Geometry check sheet. Reference: the model listing, model coordinates, mm. A direction names the side the tool comes from. Give positions to 0.01 mm unless a question says otherwise; leave off trailing zeros. Write each loop counter-clockwise with the first axis right and the second up, starting at its lowest first coordinate (ties: lowest second). Pieces come first, ordered by that corner, then holes. Notation, with made-up numbers: (76.5, -36) - (93.5, -36) arc R24 ccw to (93.5, 2) - close; hole circle Ø4 at (75, 0.5). An arc over 180 degrees is marked (long way). One line per question, with ' | ' between items. Start each with the question number.
Q1. Section check C-C on z = 5.75. Record the boundary of the cut face in (x, y) (3 decimals), and give its area (3 significant figures).
Q2. Set-up check for faces 4 (the face through (-33, 19.05, 6)), 5 (the face through (-1, 5, 0)), 6 (the face through (28.575, -4, 6)), 7 (the face through (-5.506, -24.796, 8.004)), 8 (the face through (0, -28.575, 6)): record each of +Z, -Z, +X, -X, +Y, -Y from which the full face is reachable in a straight line by a thin tool's end or side.
Q3. Thickness scan on L1, parallel to Y at x = 0, z = 8.25 (3 decimals); L2, parallel to Z at x = -16, y = 3 (3 decimals); L3, parallel to X at y = -13.5, z = 10 (3 decimals). Record the ranges inside material, lowest first. Write a range as [from, to].
Q4. Section check D-D on x = 32. Record the boundary of the cut face in (y, z), and give its area (3 significant figures).
Q5. Release check for a two-part mould opening along X. For faces 1 (the face through (-1, 27, 12.7)), 2 (the face through (38.1, 28, 6)), 3 (the face through (0, 0, 3.175)) record: +X half, -X half, draft (parallel to the pull), parting line (faces both ways), or undercut.
Q6. Section check B-B on y = 0. Record the boundary of the cut face in (x, z) (3 decimals).
Q7. Section check A-A on x = 0. Record the boundary of the cut face in (y, z) (3 decimals), and give its area (3 significant figures).
Q8. Gauge pin test, flat ends, axial feed: P1, Ø6, axis at y = -2.5, z = 7.5, coming from the +X side (3 decimals); P2, Ø3, axis at x = 33, z = 6, coming from the -Y side; P3, Ø15, axis at x = -0.5, y = -6, coming from the +Z side (3 decimals). Record the tip position at first contact, or that the pin passes through.
```python
from build123d import *

# Parameters (mm, degrees)
SKETCH1_W               = 76.2
SKETCH1_H               = 76.2
BOSS_EXTRUDE1_DEPTH     = 12.7
SKETCH2_R               = 25.4
CUT_EXTRUDE1_DEPTH      = 9.525
CUT_EXTRUDE3_DEPTH      = 1
CUT_EXTRUDE3_DEPTH_BACK = 13.7


with BuildPart() as part:
    # Sketch1 → Boss-Extrude1 (new body)
    with BuildSketch(Plane.XY):
        Rectangle(SKETCH1_W, SKETCH1_H)
    extrude(amount=BOSS_EXTRUDE1_DEPTH)

    # Sketch2 → Cut-Extrude1 (cut)
    with BuildSketch(Plane.XY.offset(12.7)):
        Circle(SKETCH2_R)
    extrude(amount=-CUT_EXTRUDE1_DEPTH, mode=Mode.SUBTRACT)

    # Sketch3 → Cut-Extrude3 (cut, two sides)
    with BuildSketch(Plane.XY.offset(12.7)) as cut_extrude3_sk:
        Polygon((238.6, 19.05), (38.1, 19.05), (28.575, 19.05), (28.575, -28.575), (-28.575, -28.575), (-28.575, 19.05), (-38.1, 19.05), (-238.6, 19.05), (-238.6, -381.95), (238.6, -381.95), align=None)
    extrude(amount=CUT_EXTRUDE3_DEPTH, mode=Mode.SUBTRACT)
    extrude(cut_extrude3_sk.sketch, amount=-CUT_EXTRUDE3_DEPTH_BACK, mode=Mode.SUBTRACT)


solid = part.part
```
Working result:
1) outline: (-38.1, 19.05) - (-28.575, 19.05) - (-28.575, -28.575) - (28.575, -28.575) - (28.575, 19.05) - (38.1, 19.05) - (38.1, 38.1) - (-38.1, 38.1) - close; hole circle Ø50.8 at (0, 0) | area: 2,150 mm2
2) face 4: +Z, -Z, -X, -Y | face 5: -Z, +X, -X, +Y, -Y | face 6: +Z, -Z, +X, -Y | face 7: +Z | face 8: +Z, -Z, +X, -X, -Y
3) L1: y = [-28.575, -25.4], [25.4, 38.1] | L2: z = [0, 3.175] | L3: x = [-28.575, -21.515], [21.515, 28.575]
4) outline: (19.05, 0) - (38.1, 0) - (38.1, 12.7) - (19.05, 12.7) - close | area: 242 mm2
5) face 1: draft | face 2: +X half | face 3: undercut
6) outline: (-28.575, 0) - (28.575, 0) - (28.575, 12.7) - (25.4, 12.7) - (25.4, 3.175) - (-25.4, 3.175) - (-25.4, 12.7) - (-28.575, 12.7) - close
7) outline: (-28.575, 0) - (38.1, 0) - (38.1, 12.7) - (25.4, 12.7) - (25.4, 3.175) - (-25.4, 3.175) - (-25.4, 12.7) - (-28.575, 12.7) - close | area: 363 mm2
8) P1: stops at x = 28.575 | P2: stops at y = 19.05 | P3: stops at z = 3.175
